Print and shaded views of the part. All mm, measured from the part's lowest x, y and z. Round coordinates to 2 decimals unless told otherwise and drop trailing zeros. Write each loop counter-clockwise with the first axis right and the second up, starting at its lowest first coordinate (ties: lowest second). Pieces come first, ordered by that corner, then holes. Notation, with made-up numbers: (82, 79) - (104, 79) arc R20 ccw to (104, 108) - close; hole circle Ø3 at (49.5, 38.5). An arc over 180 degrees is marked (long way). Put each result on its own line as item: value. Start each with the question number.
Item 1: Cut at A-A (y = 30.5). Give the cut face in (x, z) (1 decimal).
Item 2: Cut at B-B (z = 18.25). Give the cut face in (x, y) (1 decimal), and give its area (3 significant figures).
Item 3: Cut at D-D (y = 5.5). Give the cut face in (x, z) (1 decimal), and give its area (3 significant figures).
Item 4: Cut at C-C (x = 14). Give the cut face in (y, z) (1 decimal), and give its area (3 significant figures).
Item 5: Drill centre lines: line 1 (X direction, y = 21, z = 21.5) (1 decimal); line 2 (Y direction, x = 25.5, z = 12) (1 decimal); line 3 (X direction, y = 28.5, z = 20.25) (1 decimal). Where is each one in solid material? Low to high. Write a range as from..to.
Item 6: Mould opens along Y. For the marked faces 1, 2 and 3 say: released by +Y, released by -Y, zero draft, split by the parting line, or undercut.
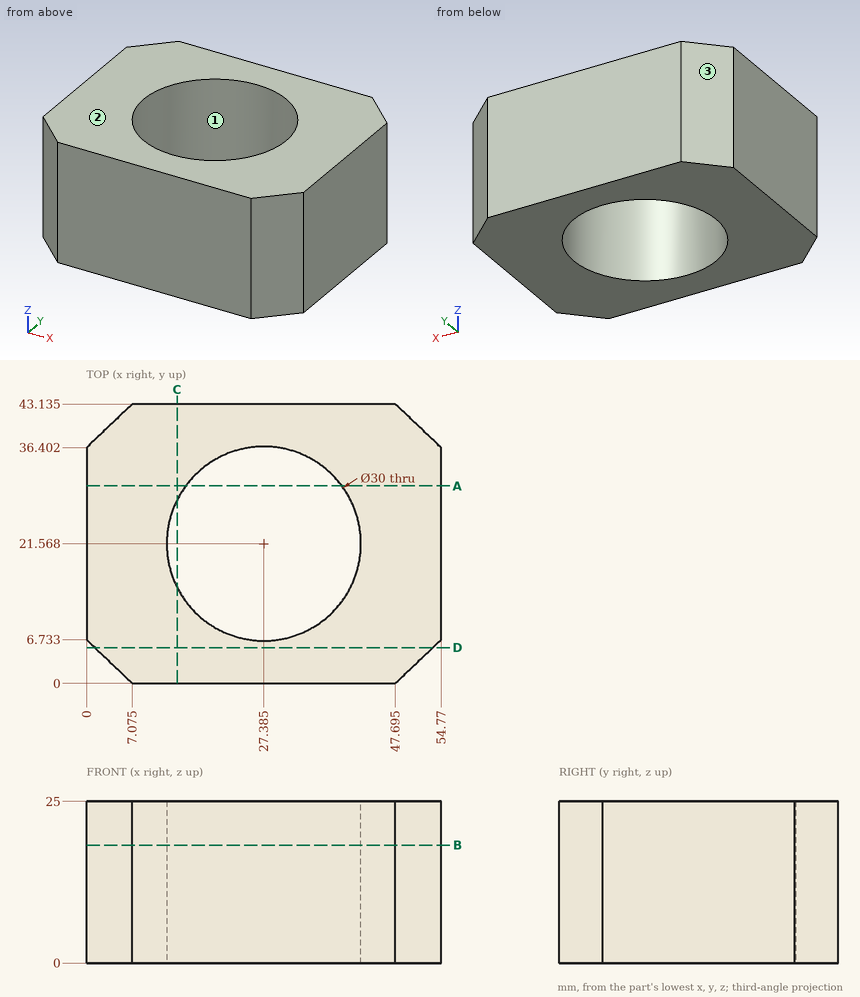
Output values:
1. outline: (0, 0) - (15.3, 0) - (15.3, 25) - (0, 25) - close; (39.4, 0) - (54.8, 0) - (54.8, 25) - (39.4, 25) - close
2. outline: (0, 6.7) - (7.1, 0) - (47.7, 0) - (54.8, 6.7) - (54.8, 36.4) - (47.7, 43.1) - (7.1, 43.1) - (0, 36.4) - close; hole circle Ø30 at (27.4, 21.6)
2. area: 1,560 mm2
3. outline: (1.3, 0) - (53.5, 0) - (53.5, 25) - (1.3, 25) - close
3. area: 1,300 mm2
4. outline: (0, 0) - (14.8, 0) - (14.8, 25) - (0, 25) - close; (28.3, 0) - (43.1, 0) - (43.1, 25) - (28.3, 25) - close
4. area: 740 mm2
5. line 1: 0..12.4, 42.4..54.8
5. line 2: 0..6.7, 36.4..43.1
5. line 3: 0..14.1, 40.7..54.8
6. face 1: undercut
6. face 2: zero draft
6. face 3: released by +Y
